Study the drawing (mm; zero at the part's minimum x, y, z) and answer. A direction names the side the tool comes from. Coordinates: 2 decimals unless noted, no trailing zeros. Write each loop counter-clockwise with the first axis right and the second up, starting at its lowest first coordinate (ties: lowest second). Pieces come first, ordered by that corner, then holes. Notation, with made-up numbers: M -34.5,10 L 3.5,10 A10 ccw 3.5,21 Z; hole C -11,76.25 d3. An arc over 180 degrees is marked long. Answer as CSV lines item,"result". Start each with the question number.
(1) A cutting plane is placed at A-A on y = 100. Give the vertices of the cut face in (x, z) (1 decimal), then the cut area to 3 significant figures.
(2) Flat-ended cylindrical pins translate along their axes: P1, Ø6, axis at x = 476, y = 162, coming from the -Z side; P2, Ø2, axis at y = 134.5, z = 49, coming from the -X side; P3, Ø2, axis at y = 62, z = 55, coming from the +X side; P4, Ø8, axis at x = 1402.5, y = 101.5, coming from the +Z side. Find the tip coordinate at first contact, or state that the pin passes through.
(3) A cutting plane is placed at D-D on y = 182. Give the vertices of the cut face in (x, z).
(4) Find the intervals of material crossed by L1, parallel to Z at x = 587, y = 120.5; L2, parallel to X at y = 106, z = 81; L3, parallel to X at y = 60.5, z = 139 (1 decimal), in increasing order. Write a range as [from, to].
(5) For the marked faces 1 and 2, determine the directions among +Z, -Z, +X, -X, +Y, -Y from which every point of the face is accessible in a straight line to the end or side of a thin tool.
(6) A cutting plane is placed at B-B on x = 1868. Give the vertices of the cut face in (y, z).
(7) A cutting plane is placed at C-C on z = 114. Give the vertices of the cut face in (x, y) (1 decimal).
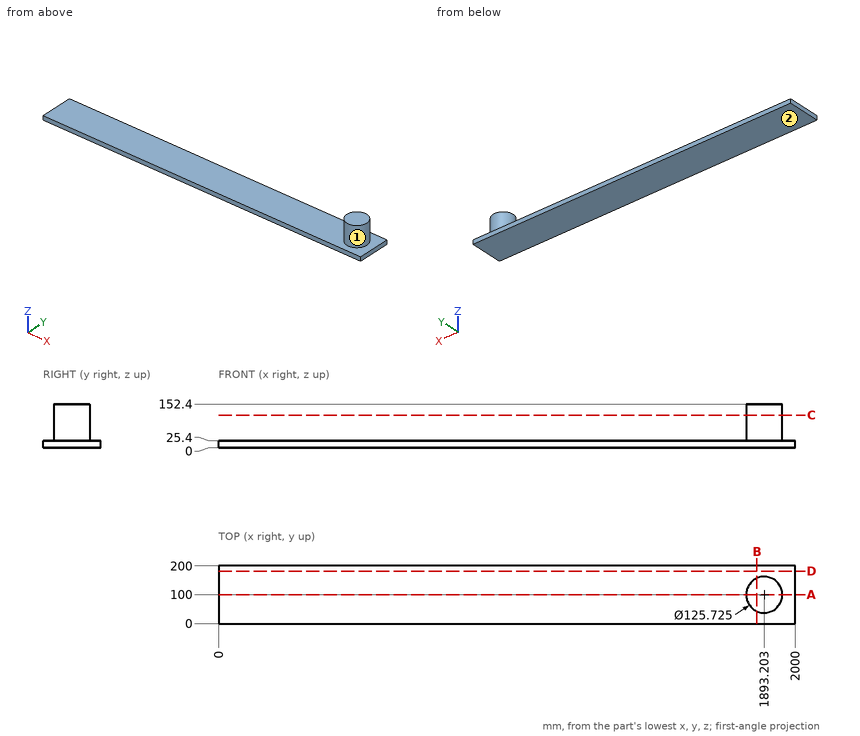
Here are the results:
1,outline,"M 0,0 L 2000,0 L 2000,25.4 L 1956.1,25.4 L 1956.1,152.4 L 1830.3,152.4 L 1830.3,25.4 L 0,25.4 Z"
1,area,"66,800 mm^2"
2,P1,"stops at z = 0"
2,P2,"stops at x = 1840.01"
2,P3,"stops at x = 1944.02"
2,P4,"stops at z = 25.4"
3,outline,"M 0,0 L 2000,0 L 2000,25.4 L 0,25.4 Z"
4,L1,"z = [0, 25.4]"
4,L2,"x = [1830.63, 1955.78]"
4,L3,"x = [1844.3, 1942.1]"
5,face 1,"+Z"
5,face 2,"-Z, +X, -X, +Y, -Y"
6,outline,"M 0,0 L 200,0 L 200,25.4 L 157.59,25.4 L 157.59,152.4 L 42.41,152.4 L 42.41,25.4 L 0,25.4 Z"
7,outline,"C 1893.2,100 d125.7"
